Here's how the part is built. I have some questions about the finished solid (model axes, mm). Face numbers are marked on the shaded views. Coordinates: 2 decimals unless noted, no trailing zeros. Write each loop counter-clockwise with the first axis right and the second up, starting at its lowest first coordinate (ties: lowest second). Pieces come first, ordered by that corner, then holes. Notation, with made-up numbers: (11, -27.5) -> (63, -27.5) arc R24 ccw to (63, 3.5) -> close; hole circle Ø10 at (33, 4). An arc over 180 degrees is marked (long way). Put each result on its own line as item: value.
```python
from build123d import *

# Parameters (mm, degrees)
BOSS_EXTRUDE1_DEPTH                                 = 9.5
CUT_EXTRUDE1_REACH                                  = 14.601
SKETCH2_R                                           = 12.8397
CSK_FOR_M2_COUNTERSUNK_FLAT_HEAD_SCREW1_D           = 2.4
CSK_FOR_M2_COUNTERSUNK_FLAT_HEAD_SCREW1_DEPTH       = 9.5
CSK_FOR_M2_COUNTERSUNK_FLAT_HEAD_SCREW1_CSINK_D     = 4.4
CSK_FOR_M2_COUNTERSUNK_FLAT_HEAD_SCREW1_CSINK_ANGLE = 90


with BuildPart() as part:
    # Sketch1 → Boss-Extrude1 (new body)
    with BuildSketch(Plane.XY):
        with BuildLine():
            Line((-16, -14.5), (16, -14.5))
            ThreePointArc((16, -14.5), (17.414213562, -13.914213562), (18, -12.5))
            Line((18, -12.5), (18, 14.5))
            Line((18, 14.5), (-18, 14.5))
            Line((-18, 14.5), (-18, -12.5))
            ThreePointArc((-18, -12.5), (-17.414213562, -13.914213562), (-16, -14.5))
        make_face()
    extrude(amount=BOSS_EXTRUDE1_DEPTH)

    # Sketch2 → Cut-Extrude1 (cut, up to next)
    with BuildSketch(Plane(origin=(0.961559067, 0, 10.990670426), x_dir=(0, 1, 0), z_dir=(0.087155743, 0, 0.996194698)), mode=Mode.PRIVATE) as cut_extrude1_sk1:
        Circle(SKETCH2_R)
    cut_extrude1_tool1 = extrude(cut_extrude1_sk1.sketch, amount=-CUT_EXTRUDE1_REACH, mode=Mode.PRIVATE) & part.part
    add(cut_extrude1_tool1.solids().sort_by_distance((0.961559, 0, 10.99067))[0], mode=Mode.SUBTRACT)

    # CSK for M2 Countersunk Flat Head Screw1
    with Locations(Plane.XY.offset(9.5)):
        with Locations((-14.7, 7), (14.7, 7)):
            CounterSinkHole(CSK_FOR_M2_COUNTERSUNK_FLAT_HEAD_SCREW1_D / 2, CSK_FOR_M2_COUNTERSUNK_FLAT_HEAD_SCREW1_CSINK_D / 2, depth=CSK_FOR_M2_COUNTERSUNK_FLAT_HEAD_SCREW1_DEPTH, counter_sink_angle=CSK_FOR_M2_COUNTERSUNK_FLAT_HEAD_SCREW1_CSINK_ANGLE)


solid = part.part
```
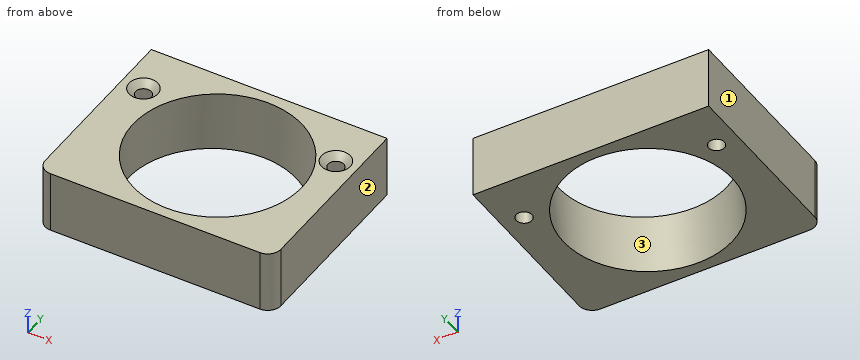
Item 1: Please list where these lines run through material, in increasing order: line 1 along Y through (x, z) = (14.7, 6.75); line 2 along X through (y, z) = (7, 4.75); line 3 along X through (y, z) = (7, 6). Write a range as from..to.
Output:
line 1: y = -14.5..5.8, 8.2..14.5
line 2: x = -18..-15.9, -13.5..-10.39, 11.22..13.5, 15.9..18
line 3: x = -18..-15.9, -13.5..-10.28, 11.33..13.5, 15.9..18
Item 2: Imagine slicing it at A-A on x = -14.7. Write out the boundary of the cut face in (y, z).
Output:
outline: (-14.5, 0) -> (5.8, 0) -> (5.8, 8.5) -> (4.8, 9.5) -> (-14.5, 9.5) -> close; (8.2, 0) -> (14.5, 0) -> (14.5, 9.5) -> (9.2, 9.5) -> (8.2, 8.5) -> close
Item 3: For P1, Ø10, axis at x = 12.5, y = -3, coming from the +Z side, with a flat end and sliding along its axis, tell me the tip position at first contact or that it passes through.
Output:
P1: stops at z = 9.5
Item 4: If we mould it in two halves opening along X, with no side actions, what happens to the marked faces 1, 2 and 3? For each: released by +X, released by -X, zero draft, split by the parting line, or undercut.
Output:
face 1: released by -X
face 2: released by +X
face 3: undercut
Item 5: Imagine slicing it at D-D on z = 7.5. State how many separate pieces and enclosed holes the cut face has, then the cut area to 3 significant figures.
Output:
separate pieces: 1
enclosed holes: 3
area: 513 mm²
Item 6: Imagine slicing it at B-B on y = 7. Write out the boundary of the cut face in (x, z), then the cut area to 3 significant figures.
Output:
outline: (-18, 0) -> (-15.9, 0) -> (-15.9, 8.5) -> (-16.9, 9.5) -> (-18, 9.5) -> close; (-13.5, 0) -> (-10.8, 0) -> (-9.97, 9.5) -> (-12.5, 9.5) -> (-13.5, 8.5) -> close; (10.8, 0) -> (13.5, 0) -> (13.5, 8.5) -> (12.5, 9.5) -> (11.64, 9.5) -> close; (15.9, 0) -> (18, 0) -> (18, 9.5) -> (16.9, 9.5) -> (15.9, 8.5) -> close
area: 89.1 mm²
Item 7: Imagine slicing it at C-C on y = -10. Write out the boundary of the cut face in (x, z), then the cut area to 3 significant figures.
Output:
outline: (-18, 0) -> (-8.08, 0) -> (-7.25, 9.5) -> (-18, 9.5) -> close; (8.08, 0) -> (18, 0) -> (18, 9.5) -> (8.92, 9.5) -> close
area: 188 mm²
